Can you work these out from the model? Positions are in its coordinate system, mm. Give positions to 0.01 mm unless a question says otherwise; leave off trailing zeros. Order: outer loops, then holes, each group sorted by start corner. A loop starts at its lowest first (then second) coordinate and runs counter-clockwise, first axis right, second up. Notation, with made-up numbers: M 11.5,28 L 42.5,28 A23 ccw 42.5,53 Z; hole C -39,46.25 d6. An arc over 180 degrees is marked long. Use a Markdown table: item, result. Add a question column.
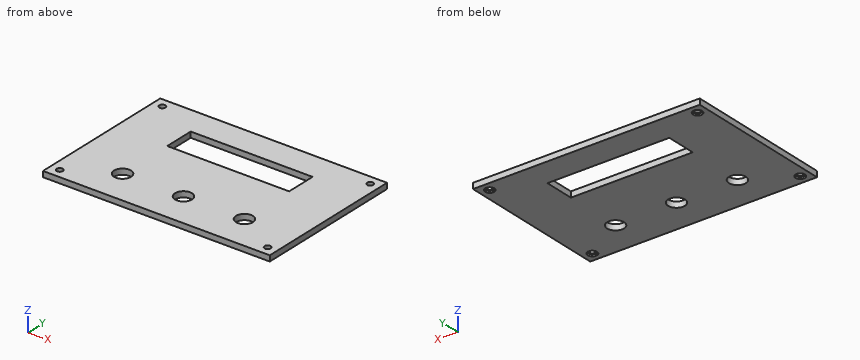
from build123d import *

# Parameters (mm, degrees)
SKICA1_W                 = 120
SKICA1_H                 = 80
P_IDAT_VYSUNUT_M3_DEPTH  = 3
SKICA1_4_OUTSIDE_W       = 150.85
SKICA1_4_OUTSIDE_H       = 110.85
SKICA1_4_OUTSIDE_W_2     = 120
SKICA1_4_OUTSIDE_H_2     = 80
SKICA1_4_OUTSIDE_R       = 4.5
SKICA1_4_OUTSIDE_W_3     = 64.5
SKICA1_4_OUTSIDE_H_3     = 16
ODEBRAT_VYSUNUT_M1_DEPTH = 3
SKICA5_R                 = 1.65
ODEBRAT_VYSUNUT_M3_DEPTH = 2
SKICA6_R                 = 2.5
ODEBRAT_VYSUNUT_M6_DEPTH = 1


with BuildPart() as part:
    # Skica1 → Přidat vysunutím3 (new body)
    with BuildSketch(Plane.XY):
        Rectangle(SKICA1_W, SKICA1_H)
    extrude(amount=P_IDAT_VYSUNUT_M3_DEPTH)

    # Skica1<4> outside → Odebrat vysunutím1 (cut)
    # profile 1 of 5: a face of its own
    with BuildSketch(Plane.XY):
        Rectangle(SKICA1_4_OUTSIDE_W, SKICA1_4_OUTSIDE_H)
        Rectangle(SKICA1_4_OUTSIDE_W_2, SKICA1_4_OUTSIDE_H_2, mode=Mode.SUBTRACT)
    # profile 2 of 5: a face of its own
    with BuildSketch(Plane.XY):
        with Locations((-32.25, -21.5)):
            Circle(SKICA1_4_OUTSIDE_R)
    # profile 3 of 5: a face of its own
    with BuildSketch(Plane.XY):
        with Locations((0, -21.5)):
            Circle(SKICA1_4_OUTSIDE_R)
    # profile 4 of 5: a face of its own
    with BuildSketch(Plane.XY):
        with Locations((32.25, -21.5)):
            Circle(SKICA1_4_OUTSIDE_R)
    # profile 5 of 5: a face of its own
    with BuildSketch(Plane.XY):
        with Locations((0, 17)):
            Rectangle(SKICA1_4_OUTSIDE_W_3, SKICA1_4_OUTSIDE_H_3)
    extrude(amount=ODEBRAT_VYSUNUT_M1_DEPTH, mode=Mode.SUBTRACT)

    # Skica5 → Odebrat vysunutím3 (cut)
    with BuildSketch(Plane.XY.offset(3)):
        with Locations((-55, 35)):
            Circle(SKICA5_R)
        with Locations((55, 35)):
            Circle(SKICA5_R)
        with Locations((-55, -35)):
            Circle(SKICA5_R)
        with Locations((55, -35)):
            Circle(SKICA5_R)
    extrude(amount=-ODEBRAT_VYSUNUT_M3_DEPTH, mode=Mode.SUBTRACT)

    # Skica6 → Odebrat vysunutím6 (cut)
    with BuildSketch(Plane.XY.offset(1)):
        with Locations((-55, 35)):
            Circle(SKICA6_R)
        with Locations((55, 35)):
            Circle(SKICA6_R)
        with Locations((55, -35)):
            Circle(SKICA6_R)
        with Locations((-55, -35)):
            Circle(SKICA6_R)
    extrude(amount=-ODEBRAT_VYSUNUT_M6_DEPTH, mode=Mode.SUBTRACT)


solid = part.part
1. If we section it at C-C, the plane x = 7.5: List the corners of the cut face in (y, z) for me, then the cut area to 3 significant figures.
2. If we section it at B-B, the plane y = -21.5: List the corners of the cut face in (x, z) for me, then the cut area to 3 significant figures.
3. If we section it at A-A, the plane y = 35: List the corners of the cut face in (x, z) for me.
4. If we section it at D-D, the plane x = 55: List the corners of the cut face in (y, z) for me, then the cut area to 3 significant figures.
5. Will these pins go through, and if not, where does the flat tip stop? pin 1 (1.5 mm diameter, centred on x = -55.5, y = 35.5, fed in from -Z); pin 2 (1.5 mm diameter, centred on x = 54, y = 34, fed in from -Z).
6. I need wall thicknesses on L1, parallel to Y at x = 55, z = 1.6; L2, parallel to Y at x = 0, z = 2.4; L3, parallel to Y at x = 9, z = 1.55. Which ranges of each line are inside material? Lowest first, please. Write a range as [from, to].
Geometry results:
| question | item | result |
|---|---|---|
| 1 | outline | M -40,0 L 9,0 L 9,3 L -40,3 Z; M 25,0 L 40,0 L 40,3 L 25,3 Z |
| 1 | area | 192 mm^2 |
| 2 | outline | M -60,0 L -36.75,0 L -36.75,3 L -60,3 Z; M -27.75,0 L -4.5,0 L -4.5,3 L -27.75,3 Z; M 4.5,0 L 27.75,0 L 27.75,3 L 4.5,3 Z; M 36.75,0 L 60,0 L 60,3 L 36.75,3 Z |
| 2 | area | 279 mm^2 |
| 3 | outline | M -60,0 L -57.5,0 L -57.5,1 L -56.65,1 L -56.65,3 L -60,3 Z; M -53.35,1 L -52.5,1 L -52.5,0 L 52.5,0 L 52.5,1 L 53.35,1 L 53.35,3 L -53.35,3 Z; M 56.65,1 L 57.5,1 L 57.5,0 L 60,0 L 60,3 L 56.65,3 Z |
| 4 | outline | M -40,0 L -37.5,0 L -37.5,1 L -36.65,1 L -36.65,3 L -40,3 Z; M -33.35,1 L -32.5,1 L -32.5,0 L 32.5,0 L 32.5,1 L 33.35,1 L 33.35,3 L -33.35,3 Z; M 36.65,1 L 37.5,1 L 37.5,0 L 40,0 L 40,3 L 36.65,3 Z |
| 4 | area | 217 mm^2 |
| 5 | pin 1 | passes through |
| 5 | pin 2 | stops at z = 1 |
| 6 | L1 | y = [-40, -36.65], [-33.35, 33.35], [36.65, 40] |
| 6 | L2 | y = [-40, -26], [-17, 9], [25, 40] |
| 6 | L3 | y = [-40, 9], [25, 40] |
